from build123d import *

# Parameters (mm, degrees)
SKETCH2_W                    = 79
SKETCH2_H                    = 105
BOSS_EXTRUDE1_DEPTH          = 3
SKETCH3_W                    = 60
SKETCH3_H                    = 70
SUPPORT_DEPTH                = 3
SKETCH4_W                    = 50
SKETCH4_H                    = 55
REMOVE_PLASTIC_DEPTH         = 3
SKETCH5_W                    = 50
SKETCH5_H                    = 25
BOSS_EXTRUDE3_DEPTH          = 5
SKETCH6_R                    = 1.2
CUT_EXTRUDE2_DEPTH           = 5
CUT_EXTRUDE2_DRAFT           = -5
CUT_EXTRUDE2_PROFILE_2_DEPTH = 5
CUT_EXTRUDE2_PROFILE_2_DRAFT = -5
CUT_EXTRUDE2_PROFILE_3_DEPTH = 5
CUT_EXTRUDE2_PROFILE_3_DRAFT = -5
CUT_EXTRUDE2_PROFILE_4_DEPTH = 5
CUT_EXTRUDE2_PROFILE_4_DRAFT = -5
CUT_EXTRUDE2_PROFILE_5_DEPTH = 5
CUT_EXTRUDE2_PROFILE_5_DRAFT = -5
SKETCH7_W                    = 29
SKETCH7_H                    = 15
BOSS_EXTRUDE4_DEPTH          = 30
BOSS_EXTRUDE5_DEPTH          = 33
SKETCH8_R                    = 4.5
SKETCH8_R_2                  = 2.5
CUT_EXTRUDE3_DEPTH           = 31
SKETCH10_W                   = 4
SKETCH10_H                   = 10
BOSS_EXTRUDE6_DEPTH          = 30
CUT_EXTRUDE4_DEPTH           = 3
CUT_EXTRUDE5_DEPTH           = 15
SKETCH13_W                   = 5
SKETCH13_H                   = 7
BOSS_EXTRUDE7_DEPTH          = 30
SKETCH14_R                   = 1.75
CUT_EXTRUDE6_DEPTH           = 20
CUT_EXTRUDE6_DRAFT           = -2
CUT_EXTRUDE6_PROFILE_2_DEPTH = 20
CUT_EXTRUDE6_PROFILE_2_DRAFT = -2
CUT_EXTRUDE6_PROFILE_3_DEPTH = 20
CUT_EXTRUDE6_PROFILE_3_DRAFT = -2
CUT_EXTRUDE6_PROFILE_4_DEPTH = 20
CUT_EXTRUDE6_PROFILE_4_DRAFT = -2
SKETCH16_W                   = 5.5
SKETCH16_H                   = 40
SLIDERS_DEPTH                = 2
SKETCH17_W                   = 71
SKETCH17_H                   = 2
BOSS_EXTRUDE9_DEPTH          = 3


with BuildPart() as part:
    # Sketch2 → Boss-Extrude1 (new body)
    with BuildSketch(Plane(origin=(0, 0, 0), x_dir=(1, 0, 0), z_dir=(0, 1, 0))):
        Rectangle(SKETCH2_W, SKETCH2_H)
    extrude(amount=BOSS_EXTRUDE1_DEPTH)

    # Sketch3 → support (add)
    with BuildSketch(Plane(origin=(0, 3, 0), x_dir=(1, 0, 0), z_dir=(0, 1, 0))):
        with Locations((0, -17.5)):
            Rectangle(SKETCH3_W, SKETCH3_H)
    extrude(amount=SUPPORT_DEPTH)

    # Sketch4 → remove plastic (cut)
    with BuildSketch(Plane(origin=(0, 6, 0), x_dir=(1, 0, 0), z_dir=(0, 1, 0))):
        with Locations((0, -25)):
            Rectangle(SKETCH4_W, SKETCH4_H)
    extrude(amount=-REMOVE_PLASTIC_DEPTH, mode=Mode.SUBTRACT)

    # Sketch5 → Boss-Extrude3 (add)
    with BuildSketch(Plane(origin=(0, 3, 0), x_dir=(1, 0, 0), z_dir=(0, 1, 0))):
        with Locations((14.5, 40)):
            Rectangle(SKETCH5_W, SKETCH5_H)
    extrude(amount=BOSS_EXTRUDE3_DEPTH)


with BuildPart() as cut_extrude2_tool:
    # Sketch6 → Cut-Extrude2 (with draft: the straight prism first)
    with BuildSketch(Plane(origin=(0, 8, 0), x_dir=(1, 0, 0), z_dir=(0, 1, 0))):
        with Locations((-1.5, 40)):
            Circle(SKETCH6_R)
    extrude(amount=-CUT_EXTRUDE2_DEPTH)
    # Cut-Extrude2: the draft: its side faces are tilted about the plane it starts from
    cut_extrude2_sides = [cut_extrude2_tool.faces().sort_by_distance(p)[0] for p in [
        (-2.7, 5.5, -40),
    ]]
    draft(cut_extrude2_sides, Plane(origin=(0, 8, 0), x_dir=(1, 0, 0), z_dir=(0, 1, 0)), CUT_EXTRUDE2_DRAFT)


with BuildPart() as part_1:
    add(part.part)

    # Cut-Extrude2: cut by cut_extrude2_tool
    add(cut_extrude2_tool.part, mode=Mode.SUBTRACT)


with BuildPart() as cut_extrude2_profile_2_tool:
    # Sketch6 → Cut-Extrude2 profile 2 (with draft: the straight prism first)
    with BuildSketch(Plane(origin=(0, 8, 0), x_dir=(1, 0, 0), z_dir=(0, 1, 0))):
        with Locations((6.5, 40)):
            Circle(SKETCH6_R)
    extrude(amount=-CUT_EXTRUDE2_PROFILE_2_DEPTH)
    # Cut-Extrude2 profile 2: the draft: its side faces are tilted about the plane it starts from
    cut_extrude2_profile_2_sides = [cut_extrude2_profile_2_tool.faces().sort_by_distance(p)[0] for p in [
        (5.3, 5.5, -40),
    ]]
    draft(cut_extrude2_profile_2_sides, Plane(origin=(0, 8, 0), x_dir=(1, 0, 0), z_dir=(0, 1, 0)), CUT_EXTRUDE2_PROFILE_2_DRAFT)


with BuildPart() as part_2:
    add(part_1.part)

    # Cut-Extrude2 profile 2: cut by cut_extrude2_profile_2_tool
    add(cut_extrude2_profile_2_tool.part, mode=Mode.SUBTRACT)


with BuildPart() as cut_extrude2_profile_3_tool:
    # Sketch6 → Cut-Extrude2 profile 3 (with draft: the straight prism first)
    with BuildSketch(Plane(origin=(0, 8, 0), x_dir=(1, 0, 0), z_dir=(0, 1, 0))):
        with Locations((14.5, 40)):
            Circle(SKETCH6_R)
    extrude(amount=-CUT_EXTRUDE2_PROFILE_3_DEPTH)
    # Cut-Extrude2 profile 3: the draft: its side faces are tilted about the plane it starts from
    cut_extrude2_profile_3_sides = [cut_extrude2_profile_3_tool.faces().sort_by_distance(p)[0] for p in [
        (13.3, 5.5, -40),
    ]]
    draft(cut_extrude2_profile_3_sides, Plane(origin=(0, 8, 0), x_dir=(1, 0, 0), z_dir=(0, 1, 0)), CUT_EXTRUDE2_PROFILE_3_DRAFT)


with BuildPart() as part_3:
    add(part_2.part)

    # Cut-Extrude2 profile 3: cut by cut_extrude2_profile_3_tool
    add(cut_extrude2_profile_3_tool.part, mode=Mode.SUBTRACT)


with BuildPart() as cut_extrude2_profile_4_tool:
    # Sketch6 → Cut-Extrude2 profile 4 (with draft: the straight prism first)
    with BuildSketch(Plane(origin=(0, 8, 0), x_dir=(1, 0, 0), z_dir=(0, 1, 0))):
        with Locations((22.5, 40)):
            Circle(SKETCH6_R)
    extrude(amount=-CUT_EXTRUDE2_PROFILE_4_DEPTH)
    # Cut-Extrude2 profile 4: the draft: its side faces are tilted about the plane it starts from
    cut_extrude2_profile_4_sides = [cut_extrude2_profile_4_tool.faces().sort_by_distance(p)[0] for p in [
        (21.3, 5.5, -40),
    ]]
    draft(cut_extrude2_profile_4_sides, Plane(origin=(0, 8, 0), x_dir=(1, 0, 0), z_dir=(0, 1, 0)), CUT_EXTRUDE2_PROFILE_4_DRAFT)


with BuildPart() as part_4:
    add(part_3.part)

    # Cut-Extrude2 profile 4: cut by cut_extrude2_profile_4_tool
    add(cut_extrude2_profile_4_tool.part, mode=Mode.SUBTRACT)


with BuildPart() as cut_extrude2_profile_5_tool:
    # Sketch6 → Cut-Extrude2 profile 5 (with draft: the straight prism first)
    with BuildSketch(Plane(origin=(0, 8, 0), x_dir=(1, 0, 0), z_dir=(0, 1, 0))):
        with Locations((30.5, 40)):
            Circle(SKETCH6_R)
    extrude(amount=-CUT_EXTRUDE2_PROFILE_5_DEPTH)
    # Cut-Extrude2 profile 5: the draft: its side faces are tilted about the plane it starts from
    cut_extrude2_profile_5_sides = [cut_extrude2_profile_5_tool.faces().sort_by_distance(p)[0] for p in [
        (29.3, 5.5, -40),
    ]]
    draft(cut_extrude2_profile_5_sides, Plane(origin=(0, 8, 0), x_dir=(1, 0, 0), z_dir=(0, 1, 0)), CUT_EXTRUDE2_PROFILE_5_DRAFT)


with BuildPart() as part_5:
    add(part_4.part)

    # Cut-Extrude2 profile 5: cut by cut_extrude2_profile_5_tool
    add(cut_extrude2_profile_5_tool.part, mode=Mode.SUBTRACT)

    # Sketch7 → Boss-Extrude4 (add)
    with BuildSketch(Plane(origin=(0, 3, 0), x_dir=(1, 0, 0), z_dir=(0, 1, 0))):
        with Locations((-25, 45)):
            Rectangle(SKETCH7_W, SKETCH7_H)
    extrude(amount=BOSS_EXTRUDE4_DEPTH)

    # Sketch9 → Boss-Extrude5 (add)
    with BuildSketch(Plane(origin=(0, 0, 0), x_dir=(1, 0, 0), z_dir=(0, 1, 0))):
        Polygon((-39.5, 52.5), (-39.5, -52.5), (-42.5, -52.5), (-42.5, 52.5), (-42.5, 55.5), (42.5, 55.5), (42.5, 52.5), (42.5, -52.5), (39.5, -52.5), (39.5, 52.5), align=None)
    extrude(amount=BOSS_EXTRUDE5_DEPTH)

    # Sketch8 → Cut-Extrude3 (cut)
    with BuildSketch(Plane.XY.offset(-37.5)):
        with Locations((-20.5, 13)):
            Circle(SKETCH8_R)
        with Locations((-34.5, 7)):
            Circle(SKETCH8_R_2)
        with Locations((-29.5, 23)):
            Circle(SKETCH8_R)
    extrude(amount=-CUT_EXTRUDE3_DEPTH, mode=Mode.SUBTRACT)

    # Sketch10 → Boss-Extrude6 (add)
    with BuildSketch(Plane(origin=(0, 3, 0), x_dir=(1, 0, 0), z_dir=(0, 1, 0))):
        with Locations((-37.5, -47.5)):
            Rectangle(SKETCH10_W, SKETCH10_H)
        with Locations((37.5, -47.5)):
            Rectangle(SKETCH10_W, SKETCH10_H)
    extrude(amount=BOSS_EXTRUDE6_DEPTH)

    # Sketch11 → Cut-Extrude4 (cut)
    with BuildSketch(Plane.XY.offset(-52.5)):
        with BuildLine():
            Line((12.5, 18), (32.5, 18))
            ThreePointArc((32.5, 18), (37.5, 13), (32.5, 8))
            Line((32.5, 8), (12.5, 8))
            ThreePointArc((12.5, 8), (7.5, 13), (12.5, 18))
        make_face()
    extrude(amount=-CUT_EXTRUDE4_DEPTH, mode=Mode.SUBTRACT)

    # Sketch12 → Cut-Extrude5 (cut)
    with BuildSketch(Plane.XY.offset(-37.5)):
        Polygon((-24.642135624, 33), (-10.5, 18.857864376), (-10.5, 33), align=None)
    extrude(amount=-CUT_EXTRUDE5_DEPTH, mode=Mode.SUBTRACT)

    # Sketch13 → Boss-Extrude7 (add)
    with BuildSketch(Plane(origin=(0, 3, 0), x_dir=(1, 0, 0), z_dir=(0, 1, 0))):
        with Locations((-37, 8.638097353)):
            Rectangle(SKETCH13_W, SKETCH13_H)
        with Locations((37, 8.638097353)):
            Rectangle(SKETCH13_W, SKETCH13_H)
    extrude(amount=BOSS_EXTRUDE7_DEPTH)


with BuildPart() as cut_extrude6_tool:
    # Sketch14 → Cut-Extrude6 (with draft: the straight prism first)
    with BuildSketch(Plane(origin=(0, 33, 0), x_dir=(1, 0, 0), z_dir=(0, 1, 0))):
        with Locations((-39, -48.5)):
            Circle(SKETCH14_R)
    extrude(amount=-CUT_EXTRUDE6_DEPTH)
    # Cut-Extrude6: the draft: its side faces are tilted about the plane it starts from
    cut_extrude6_sides = [cut_extrude6_tool.faces().sort_by_distance(p)[0] for p in [
        (-40.75, 23, 48.5),
    ]]
    draft(cut_extrude6_sides, Plane(origin=(0, 33, 0), x_dir=(1, 0, 0), z_dir=(0, 1, 0)), CUT_EXTRUDE6_DRAFT)


with BuildPart() as part_6:
    add(part_5.part)

    # Cut-Extrude6: cut by cut_extrude6_tool
    add(cut_extrude6_tool.part, mode=Mode.SUBTRACT)


with BuildPart() as cut_extrude6_profile_2_tool:
    # Sketch14 → Cut-Extrude6 profile 2 (with draft: the straight prism first)
    with BuildSketch(Plane(origin=(0, 33, 0), x_dir=(1, 0, 0), z_dir=(0, 1, 0))):
        with Locations((39, -48.5)):
            Circle(SKETCH14_R)
    extrude(amount=-CUT_EXTRUDE6_PROFILE_2_DEPTH)
    # Cut-Extrude6 profile 2: the draft: its side faces are tilted about the plane it starts from
    cut_extrude6_profile_2_sides = [cut_extrude6_profile_2_tool.faces().sort_by_distance(p)[0] for p in [
        (37.25, 23, 48.5),
    ]]
    draft(cut_extrude6_profile_2_sides, Plane(origin=(0, 33, 0), x_dir=(1, 0, 0), z_dir=(0, 1, 0)), CUT_EXTRUDE6_PROFILE_2_DRAFT)


with BuildPart() as part_7:
    add(part_6.part)

    # Cut-Extrude6 profile 2: cut by cut_extrude6_profile_2_tool
    add(cut_extrude6_profile_2_tool.part, mode=Mode.SUBTRACT)


with BuildPart() as cut_extrude6_profile_3_tool:
    # Sketch14 → Cut-Extrude6 profile 3 (with draft: the straight prism first)
    with BuildSketch(Plane(origin=(0, 33, 0), x_dir=(1, 0, 0), z_dir=(0, 1, 0))):
        with Locations((38, 8.638097353)):
            Circle(SKETCH14_R)
    extrude(amount=-CUT_EXTRUDE6_PROFILE_3_DEPTH)
    # Cut-Extrude6 profile 3: the draft: its side faces are tilted about the plane it starts from
    cut_extrude6_profile_3_sides = [cut_extrude6_profile_3_tool.faces().sort_by_distance(p)[0] for p in [
        (36.25, 23, -8.638097353),
    ]]
    draft(cut_extrude6_profile_3_sides, Plane(origin=(0, 33, 0), x_dir=(1, 0, 0), z_dir=(0, 1, 0)), CUT_EXTRUDE6_PROFILE_3_DRAFT)


with BuildPart() as part_8:
    add(part_7.part)

    # Cut-Extrude6 profile 3: cut by cut_extrude6_profile_3_tool
    add(cut_extrude6_profile_3_tool.part, mode=Mode.SUBTRACT)


with BuildPart() as cut_extrude6_profile_4_tool:
    # Sketch14 → Cut-Extrude6 profile 4 (with draft: the straight prism first)
    with BuildSketch(Plane(origin=(0, 33, 0), x_dir=(1, 0, 0), z_dir=(0, 1, 0))):
        with Locations((-38, 8.638097353)):
            Circle(SKETCH14_R)
    extrude(amount=-CUT_EXTRUDE6_PROFILE_4_DEPTH)
    # Cut-Extrude6 profile 4: the draft: its side faces are tilted about the plane it starts from
    cut_extrude6_profile_4_sides = [cut_extrude6_profile_4_tool.faces().sort_by_distance(p)[0] for p in [
        (-39.75, 23, -8.638097353),
    ]]
    draft(cut_extrude6_profile_4_sides, Plane(origin=(0, 33, 0), x_dir=(1, 0, 0), z_dir=(0, 1, 0)), CUT_EXTRUDE6_PROFILE_4_DRAFT)


with BuildPart() as part_9:
    add(part_8.part)

    # Cut-Extrude6 profile 4: cut by cut_extrude6_profile_4_tool
    add(cut_extrude6_profile_4_tool.part, mode=Mode.SUBTRACT)

    # Sketch16 → Sliders (cut)
    with BuildSketch(Plane(origin=(0, 3, 0), x_dir=(1, 0, 0), z_dir=(0, 1, 0))):
        with Locations((-32.75, -22.5)):
            Rectangle(SKETCH16_W, SKETCH16_H)
        with Locations((32.75, -22.5)):
            Rectangle(SKETCH16_W, SKETCH16_H)
    extrude(amount=-SLIDERS_DEPTH, mode=Mode.SUBTRACT)

    # Sketch17 → Boss-Extrude9 (add)
    with BuildSketch(Plane.XY.offset(52.5)):
        with Locations((0, 4)):
            Rectangle(SKETCH17_W, SKETCH17_H)
    extrude(amount=-BOSS_EXTRUDE9_DEPTH)


solid = part_9.part
Design review of the part built by this model. Coordinates are the model's own, in mm. A direction names the side the tool comes from. Round coordinates to 2 decimals unless told otherwise and drop trailing zeros. Write each loop counter-clockwise with the first axis right and the second up, starting at its lowest first coordinate (ties: lowest second). Pieces come first, ordered by that corner, then holes. Notation, with made-up numbers: (-38, -35.5) - (-3, -35.5) arc R26 ccw to (-3, -5.5) - close; hole circle Ø1 at (-20.75, 13). An arc over 180 degrees is marked (long way). Use a Markdown table: item, result. Add a question column.
1. Wall thickness on probe 1 along Z at (x, y) = (36.5, 13); probe 2 along X at (y, z) = (13.5, 45); probe 3 along X at (y, z) = (17.5, -18.5): over which ranges is each line inside the solid? List them lowest first.
2. Mouldability with a two-part tool opening along X and no side actions: class faces 1 (the face through (-42.5, 16, -2)), 2 (the face through (-3, 3, -18)), 3 (the face through (1, 0, -2)) as +X half, -X half, draft (parallel to the pull), parting line (faces both ways), or undercut.
3. For faces 4 (the face through (7.5, 12.9, -54)), 5 (the face through (-17.67, 26.03, -44.9)), 6 (the face through (-25, 18, -37.5)), list the 3-axis set-ups (+Z, -Z, +X, -X, +Y, -Y) from which the entire face can be reached by the end or side of a thin tool; tool diameter is ignored.
4. We need section C-C (x = -20.5). State the section outline as (y, z) points.
5. We need section D-D (z = 14). State the section outline as (x, y) points, then the cut area to 3 significant figures.
6. We need section B-B (x = 1). State the section outline as (y, z) points, then the cut area to 3 significant figures.
7. We need section A-A (y = 15). Count the separate pieces of the cut face and the enclosed holes in it, then the cut area to 3 significant figures.
8. Clearance check with flat-ended pins moving along their axes: pin 1 (8 mm diameter, centred on x = -8.5, y = 10.5, fed in from +Z); pin 2 (6 mm diameter, centred on x = 3.5, z = -37.5, fed in from -Y); pin 3 (1.5 mm diameter, centred on x = 13, y = 6.5, fed in from +Z); pin 4 (2.5 mm diameter, centred on x = -32, z = 50.5, fed in from +Y). State where each tip first meets the part, or that it passes through.
Output:
| question | item | result |
|---|---|---|
| 1 | probe 1 | z = -12.14 to -5.14, 42.5 to 52.5 |
| 1 | probe 2 | x = -42.5 to -35.5, 35.5 to 42.5 |
| 1 | probe 3 | x = -42.5 to -39.5, 39.5 to 42.5 |
| 2 | face 1 | -X half |
| 2 | face 2 | undercut |
| 2 | face 3 | draft |
| 3 | face 4 | +Z, -Z |
| 3 | face 5 | +Z, +Y |
| 3 | face 6 | +Y |
| 4 | outline | (0, -55.5) - (8.5, -55.5) - (8.5, -37.5) - (3, -37.5) - (3, -17.5) - (6, -17.5) - (6, -2.5) - (3, -2.5) - (3, 49.5) - (5, 49.5) - (5, 52.5) - (0, 52.5) - close; (17.5, -55.5) - (33, -55.5) - (33, -52.5) - (28.86, -52.5) - (28.86, -37.5) - (17.5, -37.5) - close |
| 5 | outline | (-42.5, 0) - (42.5, 0) - (42.5, 33) - (39.5, 33) - (39.5, 3) - (35.5, 3) - (35.5, 1) - (30, 1) - (30, 6) - (25, 6) - (25, 3) - (-25, 3) - (-25, 6) - (-30, 6) - (-30, 1) - (-35.5, 1) - (-35.5, 3) - (-39.5, 3) - (-39.5, 33) - (-42.5, 33) - close |
| 5 | area | 443 mm2 |
| 6 | outline | (0, -55.5) - (33, -55.5) - (33, -52.5) - (8, -52.5) - (8, -27.5) - (3, -27.5) - (3, -17.5) - (6, -17.5) - (6, -2.5) - (3, -2.5) - (3, 49.5) - (5, 49.5) - (5, 52.5) - (0, 52.5) - close |
| 6 | area | 590 mm2 |
| 7 | separate pieces | 3 |
| 7 | enclosed holes | 4 |
| 7 | area | 1,220 mm2 |
| 8 | pin 1 | stops at z = -27.5 |
| 8 | pin 2 | stops at y = 0 |
| 8 | pin 3 | stops at z = -2.5 |
| 8 | pin 4 | stops at y = 5 |
